Could you check a few things on this model? Use its own coordinates, in mm. A direction names the side the tool comes from. Coordinates: 2 decimals unless noted, no trailing zeros. Order: outer loops, then holes, each group sorted by start corner. A loop starts at its lowest first (then second) coordinate and runs counter-clockwise, first axis right, second up.
```python
from build123d import *

# Parameters (mm, degrees)
FILLET1_R = 12.7


with BuildPart() as part:
    # Sketch1 → Revolve1 (revolve)
    with BuildSketch(Plane.XY):
        Polygon((3.6957, -83.9978), (29.197852081, -52.50526491), (31.8135, -57.0357), (83.4517, -57.3786), (83.4517, -63.8556), (29.778956153, -63.8556), (6.978757892, -92.0115), (-83.4517, -92.0115), (-83.4517, -84.4169), align=None)
    revolve(axis=Axis((-83.4517, 0, 0), (1, 0, 0)))

    # Fillet1
    fillet1_edges = [part.edges().sort_by_distance(p)[0] for p in [
        (6.978757892, 92.0115, 0),
        (29.778956153, 63.8556, 0),
    ]]
    fillet(fillet1_edges, radius=FILLET1_R)


solid = part.part
```
Item 1: Suppose I cut it at A-A (x = 72.5). List the corners of the cut face in (y, z) for me.
Item 2: Which directions (+Z, -Z, +X, -X, +Y, -Y) give clear straight access to the entire face, cutting with the end or side of a thin tool? Please do faces 1 (the face through (59.311, -58.986, 24.457)), 2 (the face through (-83.452, -40, 75)), 3 (the face through (-39, 67, 51)).
Item 3: For pin 1 Ø1.5 at (x, z) = (41.5, -13.5) entering from +Y; pin 2 Ø6 at (x, z) = (-56.5, -12) entering from +Y; pin 3 Ø4 at (x, y) = (13.5, 55) entering from -Z, each with a flat end and sliding along its axis, tell me the tip position at first contact or that it passes through.
Item 4: I need wall thicknesses on line 1 (Z direction, x = -50, y = -51.5); line 2 (Y direction, x = -31, z = -34); line 3 (Y direction, x = -22, z = -23.5). Which ranges of each line are inside material? Lowest first, please.
Item 5: Thinking about a two-plate mould opening in Y: for faces 4 (the face through (25.017, -66.515, -20.947)), 5 (the face through (28, 11.7, 52.7)), 6 (the face through (83.452, -52.33, -23.95)), which applies, +Y half, -Y half, draft (parallel to the pull), parting line (faces both ways), or undercut?
Item 6: Suppose I cut it at B-B (x = -32). List the corners of the cut face in (y, z) for me, and give its area (3 significant figures).
Geometry results:
1. outline: circle Ø127.71 at (0, 0); hole circle Ø114.61 at (0, 0)
2. face 1: +X
2. face 2: +Z, -Z, -X, +Y, -Y
2. face 3: -X
3. pin 1: stops at y = 62.57
3. pin 2: stops at y = 91.57
3. pin 3: stops at z = -67.06
4. line 1: z = -76.25 to -66.68, 66.68 to 76.25
4. line 2: y = -85.5 to -76.99, 76.99 to 85.5
4. line 3: y = -88.96 to -80.77, 80.77 to 88.96
5. face 4: parting line
5. face 5: undercut
5. face 6: draft
6. outline: circle Ø184.02 at (0, 0); hole circle Ø168.34 at (0, 0)
6. area: 4,340 mm2
